Could you check a few things on this model? Use its own coordinates, in mm. A direction names the side the tool comes from. Round coordinates to 2 decimals unless told otherwise and drop trailing zeros. Write each loop counter-clockwise with the first axis right and the second up, starting at its lowest first coordinate (ties: lowest second). Pieces come first, ordered by that corner, then holes. Notation, with made-up numbers: (-39.75, -14) -> (-35.75, -14) arc R29 ccw to (-35.75, 14) -> close; hole circle Ø11 at (83.25, -6). An arc over 180 degrees is marked (long way). Answer in a Markdown table with one row per item. Add a question column.
```python
from build123d import *

# Parameters (mm, degrees)
SKETCH1_W           = 500
SKETCH1_H           = 500
BOSS_EXTRUDE1_DEPTH = 250
SKETCH2_W           = 500
SKETCH2_H           = 100
BOSS_EXTRUDE2_DEPTH = 350
SKETCH3_W           = 100
SKETCH3_H           = 400
BOSS_EXTRUDE3_DEPTH = 200
SKETCH4_W           = 100
SKETCH4_H           = 400
BOSS_EXTRUDE4_DEPTH = 200
SKETCH5_W           = 100
SKETCH5_H           = 150
CUT_EXTRUDE4_DEPTH  = 200
SKETCH8_W           = 100
SKETCH8_H           = 150
CUT_EXTRUDE5_DEPTH  = 200
FILLET4_R           = 30
FILLET5_R           = 30
FILLET6_R           = 30
SKETCH9_W           = 50
SKETCH9_H           = 50
BOSS_EXTRUDE5_DEPTH = 10


with BuildPart() as part:
    # Sketch1 → Boss-Extrude1 (new body, symmetric)
    with BuildSketch(Plane(origin=(0, 0, 0), x_dir=(1, 0, 0), z_dir=(0, 1, 0))):
        with Locations((-250, -250)):
            Rectangle(SKETCH1_W, SKETCH1_H)
    extrude(amount=BOSS_EXTRUDE1_DEPTH, both=True)

    # Sketch2 → Boss-Extrude2 (add)
    with BuildSketch(Plane(origin=(0, 250, 0), x_dir=(1, 0, 0), z_dir=(0, 1, 0))):
        with Locations((-250, -50)):
            Rectangle(SKETCH2_W, SKETCH2_H)
    extrude(amount=BOSS_EXTRUDE2_DEPTH)

    # Sketch3 → Boss-Extrude3 (add)
    with BuildSketch(Plane(origin=(0, 250, 0), x_dir=(1, 0, 0), z_dir=(0, 1, 0))):
        with Locations((-450, -300)):
            Rectangle(SKETCH3_W, SKETCH3_H)
    extrude(amount=BOSS_EXTRUDE3_DEPTH)

    # Sketch4 → Boss-Extrude4 (add)
    with BuildSketch(Plane(origin=(0, 250, 0), x_dir=(1, 0, 0), z_dir=(0, 1, 0))):
        with Locations((-50, -300)):
            Rectangle(SKETCH4_W, SKETCH4_H)
    extrude(amount=BOSS_EXTRUDE4_DEPTH)

    # Sketch5 → Cut-Extrude4 (cut)
    with BuildSketch(Plane.XY.offset(100)):
        with Locations((-450, 525)):
            Rectangle(SKETCH5_W, SKETCH5_H)
    extrude(amount=-CUT_EXTRUDE4_DEPTH, mode=Mode.SUBTRACT)

    # Sketch8 → Cut-Extrude5 (cut)
    with BuildSketch(Plane.XY.offset(100)):
        with Locations((-50, 525)):
            Rectangle(SKETCH8_W, SKETCH8_H)
    extrude(amount=-CUT_EXTRUDE5_DEPTH, mode=Mode.SUBTRACT)

    # Fillet4
    fillet4_edges = [part.edges().sort_by_distance(p)[0] for p in [
        (-400, 250, 300),
    ]]
    fillet(fillet4_edges, radius=FILLET4_R)

    # Fillet5
    fillet5_edges = [part.edges().sort_by_distance(p)[0] for p in [
        (-100, 250, 300),
    ]]
    fillet(fillet5_edges, radius=FILLET5_R)

    # Fillet6
    fillet6_edges = [part.edges().sort_by_distance(p)[0] for p in [
        (-108.786796564, 258.786796564, 100),
        (-400, 365, 100),
        (-100, 365, 100),
        (-250, 250, 100),
        (-391.213203436, 258.786796564, 100),
    ]]
    fillet(fillet6_edges, radius=FILLET6_R)

    # Sketch9 → Boss-Extrude5 (add)
    with BuildSketch(Plane.XZ.offset(250)):
        with Locations((-475, 475)):
            Rectangle(SKETCH9_W, SKETCH9_H)
        with Locations((-475, 25)):
            Rectangle(SKETCH9_W, SKETCH9_H)
        with Locations((-25, 25)):
            Rectangle(SKETCH9_W, SKETCH9_H)
        with Locations((-25, 475)):
            Rectangle(SKETCH9_W, SKETCH9_H)
    extrude(amount=BOSS_EXTRUDE5_DEPTH)


solid = part.part
```
(1) Suppose I cut it at A-A, the plane z = 82. Please give me the cut outline in (x, y), then the cut area to 3 significant figures.
(2) If we mould it in two halves opening along Z, with no side actions, what happens to faces 1 (the face through (-248.32, 258.555, 109.021)), 2 (the face through (-475, -260, 475)), 3 (the face through (-253, -250, 246))? For each: pulls with the +Z half, pulls with the -Z half, needs draft (parallel to the pull), parting line crosses it, or undercut.
(3) Suppose I cut it at C-C, the plane y = 267.5. Please give me the cut outline in (x, z).
(4) I need wall thicknesses on L1, parallel to X at y = 505, z = 88.5; L2, parallel to Y at x = -450, z = 343; L3, parallel to Z at x = -284, y = 364. Which ranges of each line are inside material? Lowest first, please.
(5) On a 3-axis mill with a long thin cutter (end or side, diameter ignored), from which of +Z, -Z, +X, -X, +Y, -Y can I reach the whole of each face in a straight line? I mean faces 4 (the face through (-252, 600, 49)), 5 (the face through (-391.445, 259.021, 312.41)). Say none if no direction works.
(6) Suppose I cut it at B-B, the plane x = -240.5. Please give me the cut outline in (y, z).
(7) For P1, Ø10, axis at x = -221, z = 395, coming from the -Y side; P2, Ø12, axis at x = -136, z = 200.5, coming from the +Y side, each with a flat end and sliding along its axis, tell me the tip position at first contact or that it passes through.
(8) Suppose I cut it at D-D, the plane z = 213.5. Please give me the cut outline in (x, y), then the cut area to 3 significant figures.
Response:
| question | item | result |
|---|---|---|
| 1 | outline | (-500, -250) -> (0, -250) -> (0, 450) -> (-100, 450) -> (-100, 600) -> (-400, 600) -> (-400, 450) -> (-500, 450) -> close |
| 1 | area | 395,000 mm² |
| 2 | face 1 | pulls with the +Z half |
| 2 | face 2 | needs draft |
| 2 | face 3 | undercut |
| 3 | outline | (-500, 0) -> (0, 0) -> (0, 500) -> (-102.73, 500) -> (-102.73, 130) arc R27.27 cw to (-130, 102.73) -> (-370, 102.73) arc R27.27 cw to (-397.27, 130) -> (-397.27, 500) -> (-500, 500) -> close |
| 4 | L1 | -400 to -100 |
| 4 | L2 | -250 to 450 |
| 4 | L3 | 0 to 100 |
| 5 | face 4 | +Z, -Z, +X, -X, +Y |
| 5 | face 5 | +Z, +Y |
| 6 | outline | (-250, 0) -> (600, 0) -> (600, 100) -> (280, 100) arc R30 cw to (250, 130) -> (250, 500) -> (-250, 500) -> close |
| 7 | P1 | y = -250 |
| 7 | P2 | y = 250 |
| 8 | outline | (-500, -250) -> (0, -250) -> (0, 450) -> (-100, 450) -> (-100, 280) arc R30 cw to (-130, 250) -> (-370, 250) arc R30 cw to (-400, 280) -> (-400, 450) -> (-500, 450) -> close |
| 8 | area | 290,000 mm² |
